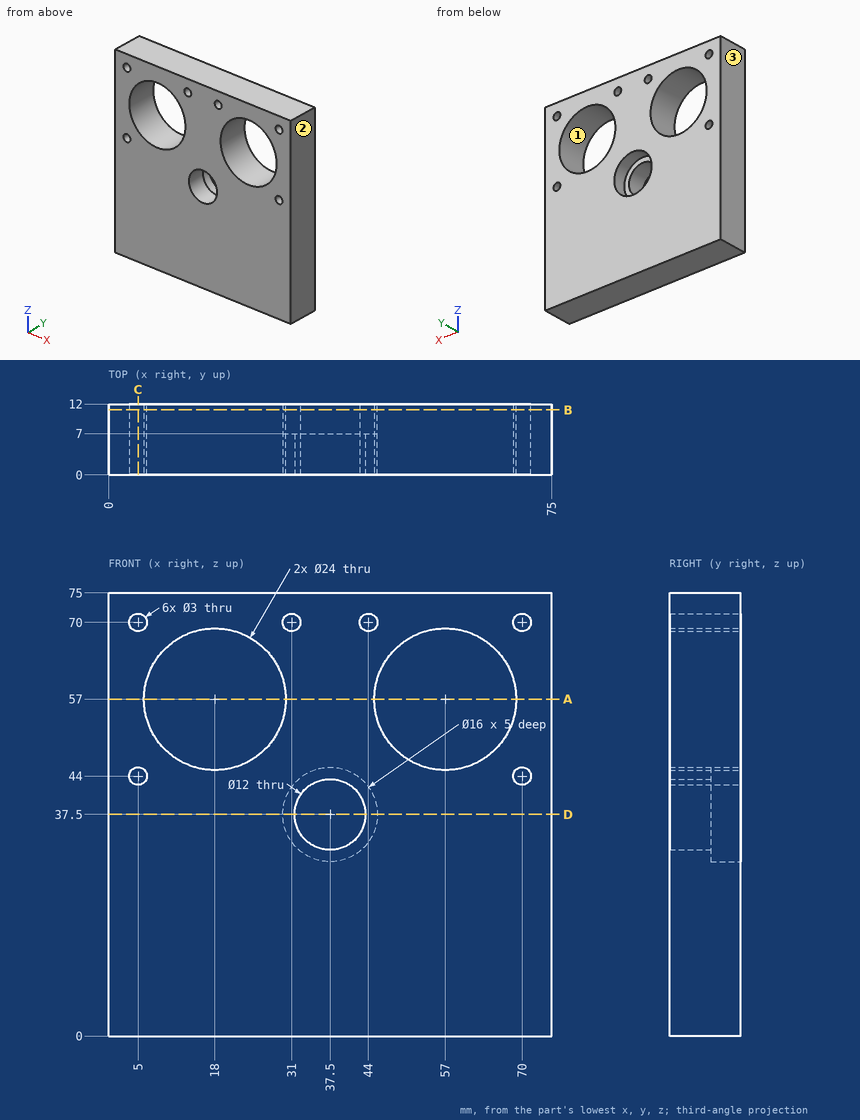
Input: dimensioned drawing with shaded views. Units: mm. Origin: part minimum x, y, z. Round coordinates to 2 decimals unless told otherwise and drop trailing zeros. Order: outer loops, then holes, each group sorted by start corner. A loop starts at its lowest first (then second) coordinate and runs counter-clockwise, first axis right, second up.
1. Cut plane D-D, the plane z = 37.5. Output: boundary loops of the cut face in (x, y).
The answers:
outline: (0, 0) - (31.5, 0) - (31.5, 7) - (29.5, 7) - (29.5, 12) - (0, 12) - close; (43.5, 0) - (75, 0) - (75, 12) - (45.5, 12) - (45.5, 7) - (43.5, 7) - close
2. Cut plane B-B, the plane y = 11. State how many separate pieces and enclosed holes the cut face has, then the cut area to 3 significant figures.
The answers:
separate pieces: 1
enclosed holes: 9
area: 4,480 mm2
3. Mould query, pull axis X, two halves, no side actions, for the marked faces 1, 2 and 3. Classes: released by +X, released by -X, zero draft, split by the parting line, or undercut.
The answers:
face 1: undercut
face 2: released by +X
face 3: released by -X
4. Pin query (flat end, axial travel): P1, Ø1.8, axis at x = 70, z = 70, coming from the -Y side; P2, Ø15.5, axis at x = 37.5, z = 37.5, coming from the +Y side. Return the tip coordinate at first contact, or that it passes through.
The answers:
P1: passes through
P2: stops at y = 7
5. Cut plane C-C, the plane x = 5. Output: boundary loops of the cut face in (y, z).
The answers:
outline: (0, 0) - (12, 0) - (12, 42.5) - (0, 42.5) - close; (0, 45.5) - (12, 45.5) - (12, 68.5) - (0, 68.5) - close; (0, 71.5) - (12, 71.5) - (12, 75) - (0, 75) - close
6. Cut plane A-A, the plane z = 57. Output: boundary loops of the cut face in (x, y).
The answers:
outline: (0, 0) - (6, 0) - (6, 12) - (0, 12) - close; (30, 0) - (45, 0) - (45, 12) - (30, 12) - close; (69, 0) - (75, 0) - (75, 12) - (69, 12) - close
7. Material intervals for line 1 (X direction, y = 6, z = 70); line 2 (Z direction, x = 70, y = 3.5); line 3 (X direction, y = 4.25, z = 65), sorted ascending.
The answers:
line 1: x = 0 to 3.5, 6.5 to 29.5, 32.5 to 42.5, 45.5 to 68.5, 71.5 to 75
line 2: z = 0 to 42.5, 45.5 to 68.5, 71.5 to 75
line 3: x = 0 to 9.06, 26.94 to 48.06, 65.94 to 75
